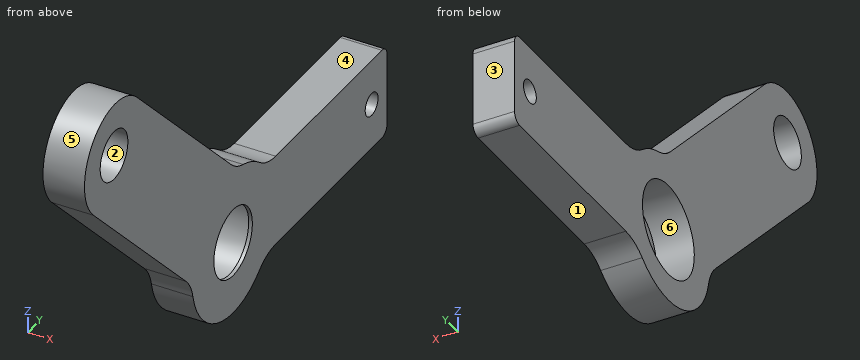
```python
from build123d import *

# Parameters (mm, degrees)
SKETCH_1_R          = 2.7
EXTRUDE_1_DEPTH     = 2.25
SKETCH_4_R          = 3.75
CUT_EXTRUDE_2_DEPTH = 5
SKETCH_7_R          = 5.05
CUT_EXTRUDE_4_DEPTH = 4.1
SKETCH_8_R          = 1.25
CUT_EXTRUDE_5_DEPTH = 6


with BuildPart() as part:
    # 草图1 → 凸台-拉伸1 (new body, symmetric)
    with BuildSketch(Plane.ZY):
        with BuildLine():
            Line((-4, 30), (4, 30))
            ThreePointArc((4, 30), (4.707106781, 29.707106781), (5, 29))
            Line((5, 29), (5, 8.306623863))
            ThreePointArc((5, 8.306623863), (5.297300284, 6.608208312), (6.153846154, 5.111768531))
            ThreePointArc((6.153846154, 5.111768531), (7.130688706, 3.626744901), (7.755507367, 1.962678138))
            ThreePointArc((7.755507367, 1.962678138), (8.255259703, 0.719581246), (9.067165566, -0.346181931))
            Line((9.067165566, -0.346181931), (27.451942184, -18.730958549))
            ThreePointArc((27.451942184, -18.730958549), (27.451942184, -27.216239924), (18.96666081, -27.216239924))
            Line((18.96666081, -27.216239924), (0.956494183, -9.206073297))
            ThreePointArc((0.956494183, -9.206073297), (-0.214644447, -8.335970475), (-1.587101368, -7.840989048))
            ThreePointArc((-1.587101368, -7.840989048), (-7.544802804, -2.660065909), (-6.153846154, 5.111768531))
            ThreePointArc((-6.153846154, 5.111768531), (-5.297300284, 6.608208312), (-5, 8.306623863))
            Line((-5, 8.306623863), (-5, 29))
            ThreePointArc((-5, 29), (-4.707106781, 29.707106781), (-4, 30))
        make_face()
        with Locations((23.452077304, -23.216375043)):
            Circle(SKETCH_1_R, mode=Mode.SUBTRACT)
    extrude(amount=EXTRUDE_1_DEPTH, both=True)

    # 草图4 → 切除-拉伸2 (cut)
    with BuildSketch(Plane.ZY.offset(-2.25)):
        Circle(SKETCH_4_R)
    extrude(amount=CUT_EXTRUDE_2_DEPTH, mode=Mode.SUBTRACT)

    # 草图7 → 切除-拉伸4 (cut)
    with BuildSketch(Plane.ZY.offset(2.25)):
        Circle(SKETCH_7_R)
    extrude(amount=-CUT_EXTRUDE_4_DEPTH, mode=Mode.SUBTRACT)

    # 草图8 → 切除-拉伸5 (cut)
    with BuildSketch(Plane(origin=(2.25, 0, 0), x_dir=(0, 0, -1), z_dir=(1, 0, 0))):
        with Locations((0, 27)):
            Circle(SKETCH_8_R)
    extrude(amount=-CUT_EXTRUDE_5_DEPTH, mode=Mode.SUBTRACT)


solid = part.part
```
Source: CAD feature listing. Evaluate the final solid. Frame: model axes, mm. Face numbers are marked on the shaded views. A direction names the side the tool comes from. Give positions to 0.01 mm unless a question says otherwise; leave off trailing zeros. Loops run counter-clockwise (first coordinate to the right, second up) from the corner with the lowest first, then second, coordinate; pieces in that order, holes last. Notation, with made-up numbers: (1.25, 22.25) -> (23.25, 22.25) arc R17 ccw to (23.25, 55.25) -> close; hole circle Ø9 at (87.25, -10). An arc over 180 degrees is marked (long way). Put each result on its own line as item: value. Start each with the question number.
1) Cut plane B-B (z = 23). Return loops of the section in (x, y), then the cut area to 3 significant figures.
2) Cut plane D-D (z = 0). Return loops of the section in (x, y).
3) Cut plane C-C (x = -0.1). Return loops of the section in (y, z), then the cut area to 3 significant figures.
4) Cut plane A-A (y = 27). Return loops of the section in (x, z), then the cut area to 4 significant figures.
5) Contact query for flat-ended pins moving along their axis: P1, Ø2, axis at y = 27, z = 0, coming from the -X side; P2, Ø2, axis at x = 0, y = 19, coming from the -Z side; P3, Ø10, axis at y = -14, z = 2, coming from the +X side. Output: stop coordinate, or through.
6) Material intervals for probe 1 along Y at (x, z) = (-1.25, 0.5); probe 2 along Z at (x, y) = (0.7, 21); probe 3 along Y at (x, z) = (2.15, 0), sorted ascending.
7) Draft query along Y for the marked faces 1, 2 and 3. Return one class per face: released by +Y, released by -Y, zero draft, split by the parting line, or undercut.
8) Reachability of the marked faces 4, 5 and 6 from +Z, -Z, +X, -X, +Y, -Y: full face, straight path, thin tool, end or side. Return the list, or none.
Results are:
1. outline: (-2.25, -28.97) -> (2.25, -28.97) -> (2.25, -25.88) -> (-2.25, -25.88) -> close; (-2.25, -20.55) -> (2.25, -20.55) -> (2.25, -14.28) -> (-2.25, -14.28) -> close
1. area: 42.2 mm2
2. outline: (-2.25, -8.46) -> (2.25, -8.46) -> (2.25, -3.75) -> (1.85, -3.75) -> (1.85, -5.05) -> (-2.25, -5.05) -> close; (-2.25, 5.05) -> (1.85, 5.05) -> (1.85, 3.75) -> (2.25, 3.75) -> (2.25, 25.75) -> (-2.25, 25.75) -> close; (-2.25, 28.25) -> (2.25, 28.25) -> (2.25, 30) -> (-2.25, 30) -> close
3. outline: (-27.22, 18.97) -> (-9.21, 0.96) arc R5 cw to (-7.84, -1.59) arc R8 ccw to (5.11, -6.15) arc R5 cw to (8.31, -5) -> (29, -5) arc R1 ccw to (30, -4) -> (30, 4) arc R1 ccw to (29, 5) -> (8.31, 5) arc R5 cw to (5.11, 6.15) arc R8 ccw to (1.96, 7.76) arc R5 cw to (-0.35, 9.07) -> (-18.73, 27.45) arc R6 ccw to start; hole circle Ø5.4 at (-23.22, 23.45); hole circle Ø10.1 at (0, 0); hole circle Ø2.5 at (27, 0)
3. area: 682 mm2
4. outline: (-2.25, -5) -> (2.25, -5) -> (2.25, -1.25) -> (-2.25, -1.25) -> close; (-2.25, 1.25) -> (2.25, 1.25) -> (2.25, 5) -> (-2.25, 5) -> close
4. area: 33.75 mm2
5. P1: passes through
5. P2: stops at z = -5
5. P3: stops at x = 2.25
6. probe 1: y = -8.8 to -5.03, 5.03 to 25.85, 28.15 to 30
6. probe 2: z = -5 to 5
6. probe 3: y = -8.46 to -3.75, 3.75 to 25.75, 28.25 to 30
7. face 1: zero draft
7. face 2: undercut
7. face 3: released by +Y
8. face 4: +Z, +X, -X, +Y
8. face 5: +X, -X
8. face 6: -X
